from build123d import *

# Parameters (mm, degrees)
SKETCH1_R           = 5
BOSS_EXTRUDE1_DEPTH = 4
SKETCH2_W           = 30
SKETCH2_H           = 38
BOSS_EXTRUDE2_DEPTH = 5
SKETCH4_W           = 30
SKETCH4_H           = 25
SKETCH4_R           = 1.6
BOSS_EXTRUDE3_DEPTH = 5
RIB1_REACH          = 77.326
SKETCH5_WALL_W      = 184.007294544
SKETCH5_WALL_H      = 5


with BuildPart() as part:
    # Sketch1 → Boss-Extrude1 (new body)
    with BuildSketch(Plane.XY):
        with BuildLine():
            Line((15, 0), (15, -40))
            Line((15, -40), (-15, -40))
            Line((-15, -40), (-15, 0))
            ThreePointArc((-15, 0), (0, 15), (15, 0))
        make_face()
        Circle(SKETCH1_R, mode=Mode.SUBTRACT)
    extrude(amount=BOSS_EXTRUDE1_DEPTH)

    # Sketch2 → Boss-Extrude2 (add)
    with BuildSketch(Plane.XZ.offset(40)):
        with Locations((0, -19)):
            Rectangle(SKETCH2_W, SKETCH2_H)
    extrude(amount=-BOSS_EXTRUDE2_DEPTH)

    # Sketch4 → Boss-Extrude3 (add)
    with BuildSketch(Plane(origin=(0, 0, -38), x_dir=(-1, 0, 0), z_dir=(0, 0, -1))):
        with Locations((0, -47.5)):
            Rectangle(SKETCH4_W, SKETCH4_H)
        with Locations((9, -50)):
            Circle(SKETCH4_R, mode=Mode.SUBTRACT)
        with Locations((-9, -50)):
            Circle(SKETCH4_R, mode=Mode.SUBTRACT)
    extrude(amount=BOSS_EXTRUDE3_DEPTH)

    # Sketch5 wall → Rib1 (add, up to next)
    with BuildSketch(Plane(origin=(0, -47.446002706, -24.203370922), x_dir=(0, 0.474942623165, 0.880016763875), z_dir=(0, -0.880016763875, 0.474942623165)), mode=Mode.PRIVATE) as rib1_sk1:
        Rectangle(SKETCH5_WALL_W, SKETCH5_WALL_H)
    rib1_tool1 = extrude(rib1_sk1.sketch, amount=-RIB1_REACH, mode=Mode.PRIVATE) - part.part
    add(rib1_tool1.solids().sort_by_distance((0, -47.446002706, -24.203370922))[0])


solid = part.part
Verification items for the finished model (mm, model axes). A direction names the side the tool comes from. Give positions to 0.01 mm unless a question says otherwise; leave off trailing zeros. Loops run counter-clockwise (first coordinate to the right, second up) from the corner with the lowest first, then second, coordinate; pieces in that order, holes last.
1) Sectioned sample at A-A, the plane x = 9. Enter the section's corners in (y, z), then the cut area to 3 significant figures.
2) Sectioned sample at C-C, the plane z = -32.5. Enter the section's corners in (x, y), then the cut area to 3 significant figures.
3) Draft check along Y on faces 1 (the cylindrical face through (0, 15, 2)), 2 (the flat face through (-15, -37, -19)), 3 (the cylindrical face through (-1.08, -4.88, 1.97)). Enter one of: pulls with the +Y half, pulls with the -Y half, needs draft (parallel to the pull), parting line crosses it, or undercut.
4) Depth check by flat-ended pin: pin 1 Ø3.5 at (x, y) = (-9, -50) entering from +Z; pin 2 Ø8 at (x, y) = (0, 0) entering from +Z; pin 3 Ø16.5 at (y, z) = (-50.5, -27) entering from -X; pin 4 Ø16 at (x, y) = (1, -50) entering from +Z. Enter the tip coordinate at first touch or a pass-through.
5) Sectioned sample at B-B, the plane y = -2. Enter the section's corners in (x, z), then the cut area to 3 significant figures.
6) Thickness scan on line 1 along Y through (x, z) = (0, 3.05); line 2 along Z through (x, y) = (12.25, 5.5); line 3 along Y through (x, z) = (-1.25, -3.5). Record the ranges inside material, lowest first.
7) Sectioned sample at D-D, the plane x = 0. Enter the section's corners in (y, z), then the cut area to 3 significant figures.
8) Set-up check for faces 4 (the flat face through (-2.5, -46, -29)), 5 (the flat face through (0, -10, 0)), 6 (the flat face through (4, -50, -38)), 7 (the flat face through (2.5, -46, -29)): record each of +Z, -Z, +X, -X, +Y, -Y from which the full face is reachable in a straight line by a thin tool's end or side.
Answers:
1. outline: (-60, -43) - (-51.6, -43) - (-51.6, -38) - (-60, -38) - close; (-48.4, -43) - (-35, -43) - (-35, 0) - (12, 0) - (12, 4) - (-40, 4) - (-40, -38) - (-48.4, -38) - close
1. area: 507 mm2
2. outline: (-15, -40) - (-2.5, -40) - (-2.5, -51.92) - (2.5, -51.92) - (2.5, -40) - (15, -40) - (15, -35) - (-15, -35) - close
2. area: 210 mm2
3. face 1: pulls with the +Y half
3. face 2: needs draft
3. face 3: undercut
4. pin 1: stops at z = -38
4. pin 2: passes through
4. pin 3: stops at x = -2.5
4. pin 4: stops at z = -14.11
5. outline: (-15, 0) - (-4.58, 0) - (-4.58, 4) - (-15, 4) - close; (4.58, 0) - (15, 0) - (15, 4) - (4.58, 4) - close
5. area: 83.3 mm2
6. line 1: y = -40 to -5, 5 to 15
6. line 2: z = 0 to 4
6. line 3: y = -40 to -35
7. outline: (-60, -43) - (-35, -43) - (-35, 0) - (-5, 0) - (-5, 4) - (-40, 4) - (-40, -10.41) - (-54.89, -38) - (-60, -38) - close; (5, 0) - (15, 0) - (15, 4) - (5, 4) - close
7. area: 700 mm2
8. face 4: +Z, -X, -Y
8. face 5: -Z, +X, -X, +Y
8. face 6: +Z, -Y
8. face 7: +Z, +X, -Y
